The model under review builds one solid part; all positions refer to its coordinate system, in mm. A direction names the side the tool comes from. Give positions to 0.01 mm unless a question says otherwise; leave off trailing zeros. Order: outer loops, then holes, each group sorted by start corner. A loop starts at its lowest first (then second) coordinate and runs counter-clockwise, first axis right, second up. Notation, with made-up numbers: M 8.5,85.25 L 20.5,85.25 A21 ccw 20.5,104.25 Z; hole C 68,39 d9. An arc over 180 degrees is marked long. One line per question, with ' | ' between items. Start each with the question number.
1. Insertion check: P1, Ø1.9, axis at x = 0, y = 60.5, coming from the -Z side; P2, Ø1.5, axis at x = 0.5, z = 0, coming from the -Y side; P3, Ø1, axis at y = 50, z = -0.5, coming from the +X side; P4, Ø3, axis at y = -35.5, z = -2.5, coming from the -X side. Each pin has a flat end and moves straight along its axis. Give the tip position at first contact, or say it passes through.
2. For faces 4 (the face through (-0.417, -56.827, 3.606)), 5 (the face through (0.31, 62.38, -0.04)), list the 3-axis set-ups (+Z, -Z, +X, -X, +Y, -Y) from which the entire face can be reached by the end or side of a thin tool; tool diameter is ignored.
3. We need section B-B on y = 44.5. Write out the cut boundary in (x, z).
4. We need section A-A on y = 60. Write out the cut boundary in (x, z), then the cut area to 3 significant figures.
5. Wall thickness on L1, parallel to Y at x = 0, z = 3.55; L2, parallel to Y at x = 0, z = 1.5; L3, parallel to Y at x = 1, z = 2: over which ranges is each line inside the solid? List them lowest first.
6. The part is to be moulded in two halves that separate along X. For faces 1 (the face through (0.417, 63.173, -3.606)), 2 (the face through (0.417, -56.827, -3.606)), 3 (the face through (-0.47, 63.57, 0.06)), say which applies: +X half, -X half, draft (parallel to the pull), parting line (faces both ways), or undercut.
Autodesk Inventor part; units mm, degrees
ref_plane "YZ Plane" through (0, 0, 0) normal (1, 0, 0) x (0, 1, 0)
ref_plane "XZ Plane" through (0, 0, 0) normal (0, 1, 0) x (-1, 0, 0)
ref_plane "XY Plane" through (0, 0, 0) normal (0, 0, 1) x (1, 0, 0)
sketch "Sketch2" plane through (0, 0, 0) normal (0, 1, 0) x (-1, 0, 0)
  circle A0 centre (0, 0) radius 2.4 construction
  line L0 (-0.8, 2.2627) -> (-0.8, 0.8)
  line L1 (-0.8, 0.8) -> (-2.2627, 0.8)
  line L2 (-2.2627, -0.8) -> (-0.8, -0.8)
  line L3 (-0.8, -0.8) -> (-0.8, -2.2627)
  line L4 (0.8, -2.2627) -> (0.8, -0.8)
  line L5 (0.8, -0.8) -> (2.2627, -0.8)
  line L6 (2.2627, 0.8) -> (0.8, 0.8)
  line L7 (0.8, 0.8) -> (0.8, 2.2627)
  arc A1 (0.8, 2.2627) -> (-0.8, 2.2627) centre (0, 0) ccw
  arc A2 (-2.2627, 0.8) -> (-2.2627, -0.8) centre (0, 0) ccw
  arc A3 (-0.8, -2.2627) -> (0.8, -2.2627) centre (0, 0) ccw
  arc A4 (2.2627, -0.8) -> (2.2627, 0.8) centre (0, 0) ccw
  dimension "d1" = 4.8
  dimension "d0" = 1.6
extrude "Extrusion1" add sketch "Sketch2" along normal mid plane 120
sketch "Sketch3" plane through (0, 0, 0) normal (0, 0, 1) x (1, 0, 0)
  line L0 (0.8, 60) -> (-0.8, 60)
  line L1 (-0.8, -60) -> (0.8, -60)
  circle A0 centre (0, 60) radius 3.6
  circle A1 centre (0, 60) radius 2.4
  circle A2 centre (0, -60) radius 3.6
  circle A3 centre (0, -60) radius 2.4
  point P0 (0, 0)
  dimension "d4" = 7.2
  dimension "d5" = 4.8
extrude "Extrusion2" add sketch "Sketch3" along normal mid plane 8 contours A0 | A1 | A2 | A3
sketch "Sketch4" plane through (0, 60, -4) normal (0, 0, -1) x (-1, 0, 0)
  circle A0 centre (0, 0) radius 3.6
  circle A1 centre (0, 0) radius 2.4
  circle A2 centre (0, -120) radius 3.6
  circle A3 centre (0, -120) radius 2.4
  point P0 (0, -3.6)
  point P1 (0, -60)
  dimension "d10" = 4.8
extrude "Extrusion4" cut sketch "Sketch4" against normal through all contours A1 | A3
sketch "Skizze6" plane through (0, 60, -4) normal (0, 0, -1) x (-1, 0, 0)
  circle A0 centre (0, 0) radius 2.4
  circle A1 centre (0, 0) radius 3.6
  circle A2 centre (0, 0) radius 3.2
  point P0 (0, -60)
  dimension "d26" = 6.4
extrude "Extrusion5" cut sketch "Skizze6" against normal blind 0.8 contours A2
pattern_circular "Circular Pattern1" count 2 over 360 about axis through (0, 0, 0) along (0, -1, 0) of "Extrusion5"
pattern_linear "Rectangular Pattern1" count 2 spacing 120 along (0, -1, 0) of "Circular Pattern1", "Extrusion5"
equation "\"d1\" = kd"
equation "\"d0\" = axlet"
equation "\"d2\" = 15 * lu"
equation "\"d4\" = tlad"
equation "\"d5\" = tpd"
equation "\"d6\" = lu"
equation "\"d10\" = tpd"
equation "\"d11\" = tsl"
equation "\"d26\" = tsd"
equation "\"d27\" = tsl"
equation "\"d25\" = 15 * lu"
properties part number "2739a-Black" material "ABS Plastic"
Entries:
1) P1: passes through | P2: stops at y = -63.6 | P3: stops at x = 2.4 | P4: stops at x = -0.8
2) face 4: +Z | face 5: +Z, -Z
3) outline: M -2.26,-0.8 L -0.8,-0.8 L -0.8,-2.26 A2.4 ccw 0.8,-2.26 L 0.8,-0.8 L 2.26,-0.8 A2.4 ccw 2.26,0.8 L 0.8,0.8 L 0.8,2.26 A2.4 ccw -0.8,2.26 L -0.8,0.8 L -2.26,0.8 A2.4 ccw Z
4) outline: M -3.6,-4 L -3.2,-4 L -3.2,-3.2 L -2.4,-3.2 L -2.4,3.2 L -3.2,3.2 L -3.2,4 L -3.6,4 Z; M 2.4,-3.2 L 3.2,-3.2 L 3.2,-4 L 3.6,-4 L 3.6,4 L 3.2,4 L 3.2,3.2 L 2.4,3.2 Z | area: 16.6 mm^2
5) L1: y = -63.6 to -63.2, -56.8 to -56.4, 56.4 to 56.8, 63.2 to 63.6 | L2: y = -63.6 to -62.4, -57.6 to 57.6, 62.4 to 63.6 | L3: y = -63.46 to -62.18, -57.82 to -56.54, 56.54 to 57.82, 62.18 to 63.46
6) face 1: undercut | face 2: undercut | face 3: parting line
